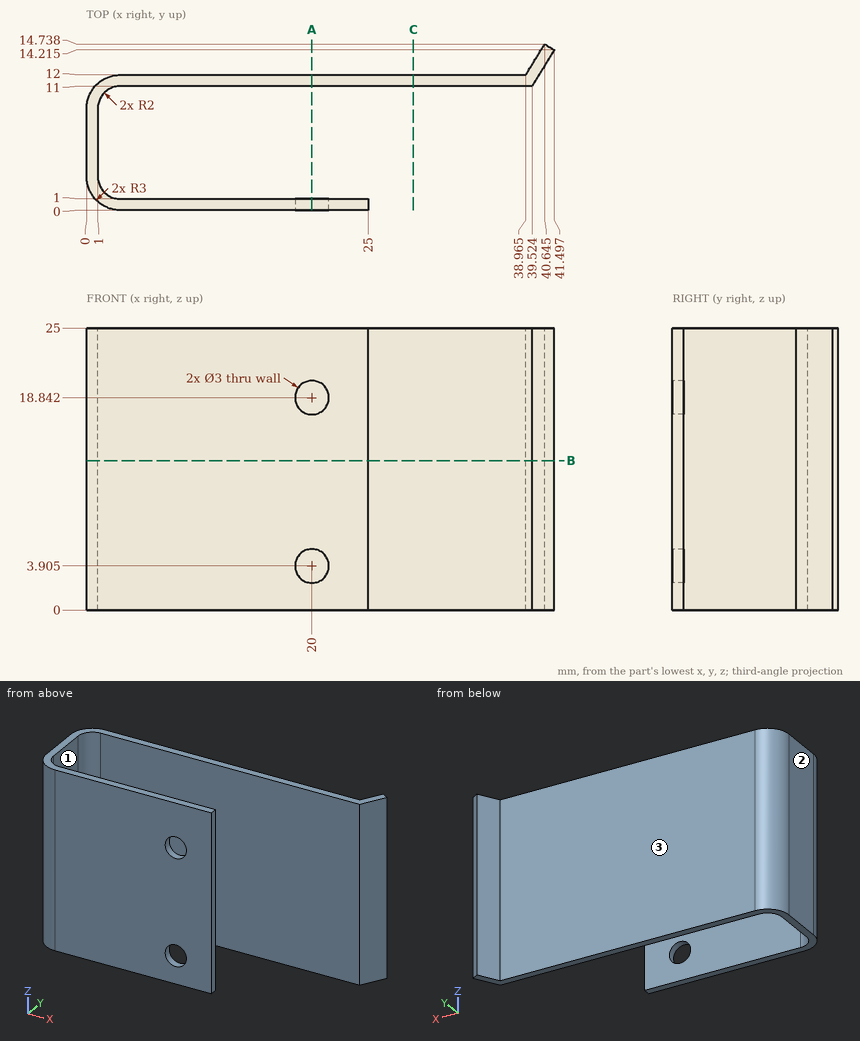
Verification items for this drawing (mm, ordinates from the low corner). A direction names the side the tool comes from. Coordinates: 2 decimals unless noted, no trailing zeros. Loops run counter-clockwise (first coordinate to the right, second up) from the corner with the lowest first, then second, coordinate; pieces in that order, holes last.
Item 1: Sectioned sample at A-A, the plane x = 20. Record the boundary of the cut face in (y, z) (1 decimal).
Item 2: Go/stop test with flat-tipped pins: pin 1 Ø0.5 at (y, z) = (0.5, 13.5) entering from +X; pin 2 Ø12.5 at (x, z) = (29, 9) entering from +Y; pin 3 Ø1 at (y, z) = (6.5, 15) entering from +X. Record where each tip stops, or that it passes through.
Item 3: Access from +Z, -Z, +X, -X, +Y, -Y to the whole of each face (thin tool, end or side, straight path). Record for the marked faces 1, 2 and 3.
Item 4: Sectioned sample at C-C, the plane x = 29. Record the boundary of the cut face in (y, z), then the cut area to 3 significant figures.
Item 5: Thickness scan on line 1 (Z direction, x = 20, y = 0.5) (1 decimal); line 2 (Y direction, x = 8, z = 5.75); line 3 (Z direction, x = 19, y = 0.5) (1 decimal). Record the ranges inside material, lowest first.
Item 6: Sectioned sample at B-B, the plane z = 13.25. Record the boundary of the cut face in (x, y) (1 decimal).
Check result:
1. outline: (0, 0) - (1, 0) - (1, 2.4) - (0, 2.4) - close; (0, 5.4) - (1, 5.4) - (1, 17.3) - (0, 17.3) - close; (0, 20.3) - (1, 20.3) - (1, 25) - (0, 25) - close; (11, 0) - (12, 0) - (12, 25) - (11, 25) - close
2. pin 1: stops at x = 25
2. pin 2: stops at y = 12
2. pin 3: stops at x = 1
3. face 1: +Z, -Z, +X
3. face 2: +Z, -Z, -X, +Y, -Y
3. face 3: +Z, -Z, -X, +Y
4. outline: (11, 0) - (12, 0) - (12, 25) - (11, 25) - close
4. area: 25.0 mm2
5. line 1: z = 0 to 2.4, 5.4 to 17.3, 20.3 to 25
5. line 2: y = 0 to 1, 11 to 12
5. line 3: z = 0 to 2.8, 5 to 17.7, 20 to 25
6. outline: (0, 3) arc R3 ccw to (3, 0) - (25, 0) - (25, 1) - (3, 1) arc R2 cw to (1, 3) - (1, 9) arc R2 cw to (3, 11) - (39.5, 11) - (41.5, 14.2) - (40.6, 14.7) - (39, 12) - (3, 12) arc R3 ccw to (0, 9) - close
